Source: CAD feature listing. Evaluate the final solid. Frame: model axes, mm. A direction names the side the tool comes from. Give positions to 0.01 mm unless a question says otherwise; leave off trailing zeros. Loops run counter-clockwise (first coordinate to the right, second up) from the corner with the lowest first, then second, coordinate; pieces in that order, holes last. Notation, with made-up numbers: M 9.25,58 L 41.25,58 A19 cw 41.25,74 Z; hole C 87.5,36.5 d11. An arc over 180 degrees is marked long. Answer in a Markdown table with one row per item.
```python
from build123d import *

# Parameters (mm, degrees)
F0_W     = 330.2
F0_H     = 228.6
F1_DEPTH = 12.7
F3_DEPTH = 241.3
F5_DEPTH = 12.7
F6_W     = 50.8
F6_H     = 12.7
F7_DEPTH = 12.7
F8_W     = 50.8
F8_H     = 12.7
F9_DEPTH = 12.7


with BuildPart() as f1:
    # F0 (on Front) → F1 (new body)
    with BuildSketch(Plane.XZ):
        Rectangle(F0_W, F0_H)
    extrude(amount=F1_DEPTH)

    # F2 (on face) → F3 (join)
    with BuildSketch(Plane.XZ.offset(12.7)):
        Polygon((-162.56, -111.76), (-162.56, 114.3), (-165.1, 114.3), (-165.1, -114.3), (165.1, -114.3), (165.1, 114.3), (162.56, 114.3), (162.56, -111.76), align=None)
    extrude(amount=F3_DEPTH)

    # F4 (on face) → F5 (join)
    with BuildSketch(Plane.XZ.offset(254)):
        Polygon((-162.56, 114.3), (-165.1, 114.3), (-165.1, -114.3), (165.1, -114.3), (165.1, 114.3), align=None)
    extrude(amount=F5_DEPTH)

    # F6 (on face) → F7 (join)
    with BuildSketch(Plane.XZ.offset(266.7)):
        with Locations((0, 120.65)):
            Rectangle(F6_W, F6_H)
        with Locations((0, 107.95)):
            Rectangle(F6_W, F6_H)
    extrude(amount=F7_DEPTH)

    # F8 (on face) → F9 (join)
    with BuildSketch(Plane(origin=(0, 0, 0), x_dir=(-1, 0, 0), z_dir=(0, 1, 0))):
        with Locations((0, 107.95)):
            Rectangle(F8_W, F8_H)
        with Locations((0, 120.65)):
            Rectangle(F8_W, F8_H)
    extrude(amount=F9_DEPTH)


solid = f1.part
```
1) Section A-A, the plane z = -43.5. Return loops of the section in (x, y).
Reply:
| item | result |
|---|---|
| outline | M -165.1,-266.7 L 165.1,-266.7 L 165.1,0 L -165.1,0 Z; hole M -162.56,-254 L 162.56,-254 L 162.56,-12.7 L -162.56,-12.7 Z |
2) Section C-C, the plane y = -211.5. Return loops of the section in (x, z), then the cut area to 3 significant figures.
Reply:
| item | result |
|---|---|
| outline | M -165.1,-114.3 L 165.1,-114.3 L 165.1,114.3 L 162.56,114.3 L 162.56,-111.76 L -162.56,-111.76 L -162.56,114.3 L -165.1,114.3 Z |
| area | 1,990 mm² |
3) Material intervals for L1, parallel to Y at x = -87.5, z = -63; L2, parallel to X at y = -155, z = -87; L3, parallel to Z at x = -147, y = -262, sorted ascending.
Reply:
| item | result |
|---|---|
| L1 | y = -266.7 to -254, -12.7 to 0 |
| L2 | x = -165.1 to -162.56, 162.56 to 165.1 |
| L3 | z = -114.3 to 114.3 |
4) Set-up query: faces 1 (the flat face through (25.4, -273, 114)), 2 (the flat face through (0, 6, 101.6)), 3 (the flat face through (0, -273, 101.6)), 4 (the flat face through (25.4, 6, 114)), 5 (the flat face through (1, -4, 114.3)). Return all of +Z, -Z, +X, -X, +Y, -Y with unobstructed straight access to the full face (end or side cutting, diameter ignored); none if empty.
Reply:
| item | result |
|---|---|
| face 1 | +Z, -Z, +X, -Y |
| face 2 | -Z, +X, -X, +Y |
| face 3 | -Z, +X, -X, -Y |
| face 4 | +Z, -Z, +X, +Y |
| face 5 | +Z, +X, -X |
5) Pin query (flat end, axial travel): pin 1 Ø12 at (x, z) = (-109.5, -14) entering from +Y; pin 2 Ø10 at (x, y) = (5.5, 4) entering from -Z; pin 3 Ø8 at (x, y) = (-124, -124) entering from +Z; pin 4 Ø10 at (y, z) = (-270.5, 119) entering from -X. Return the tip coordinate at first contact, or that it passes through.
Reply:
| item | result |
|---|---|
| pin 1 | stops at y = 0 |
| pin 2 | stops at z = -114.3 |
| pin 3 | stops at z = -111.76 |
| pin 4 | stops at x = -25.4 |
6) Section B-B, the plane x = 98. Return loops of the section in (y, z), then the cut area to 3 significant figures.
Reply:
| item | result |
|---|---|
| outline | M -266.7,-114.3 L 0,-114.3 L 0,114.3 L -12.7,114.3 L -12.7,-111.76 L -254,-111.76 L -254,114.3 L -266.7,114.3 Z |
| area | 6,420 mm² |
7) Pull-direction query (X, two-part tool) for faces 6 (the flat face through (-2, -131, -114.3)), 7 (the flat face through (-162.56, -132, 0)), 8 (the flat face through (-25.4, 6, 114)); classes: released by +X, released by -X, zero draft, split by the parting line, or undercut.
Reply:
| item | result |
|---|---|
| face 6 | zero draft |
| face 7 | undercut |
| face 8 | released by -X |
8) Section D-D, the plane x = 2. Return loops of the section in (y, z).
Reply:
| item | result |
|---|---|
| outline | M -279.4,101.6 L -266.7,101.6 L -266.7,-114.3 L 0,-114.3 L 0,101.6 L 12.7,101.6 L 12.7,127 L 0,127 L 0,114.3 L -12.7,114.3 L -12.7,-111.76 L -254,-111.76 L -254,114.3 L -266.7,114.3 L -266.7,127 L -279.4,127 Z |
